Work out the finished part from the listing and answer in its coordinate system (mm). A direction names the side the tool comes from. Round coordinates to 2 decimals unless told otherwise and drop trailing zeros. Write each loop counter-clockwise with the first axis right and the second up, starting at its lowest first coordinate (ties: lowest second). Pieces come first, ordered by that corner, then holes.
1. Find section B-B (y = 3.75). Write down the section's boundary in (x, z).
2. Flat-ended cylindrical pins translate along their axes: pin 1 Ø0.6 at (x, z) = (-7.5, 0) entering from -Y; pin 2 Ø0.6 at (x, z) = (-6, -0.5) entering from +Y. Find the tip coordinate at first contact, or state that the pin passes through.
3. Find section D-D (y = 0). Write down the section's boundary in (x, z), and give its area (3 significant figures).
4. Find section C-C (z = 0.2). Write down the section's boundary in (x, y), and give its area (3 significant figures).
5. Find section A-A (x = 0). Write down the section's boundary in (y, z).
6. Determine the mould class of faces 1 (the face through (4, 0, 1)), 2 (the face through (0, 6, 0)), 3 (the face through (10, 0, 0)) for opening direction Y: pulls with the +Y half, pulls with the -Y half, needs draft (parallel to the pull), parting line crosses it, or undercut.
7. A tool of negligible diameter and unlimited length cuts with its end or side. For faces 4 (the face through (4, 0, -1)), 5 (the face through (3.37, 0, 0)), 6 (the face through (-6, 3.37, 0)), from which of +Z, -Z, +X, -X, +Y, -Y can it reach the whole face along a straight path? Write none if from no direction.
8. Straight lines are drawn through the part: probe 1 along Y at (x, z) = (-3, -0.55); probe 2 along Y at (x, z) = (-6, 0); probe 3 along X at (y, z) = (4, -0.2). For each, find the intervals that lie inside material, in ascending order.
```python
from build123d import *

# Parameters (mm, degrees)
SCHIZZO1_R                   = 10
ESTRUSIONE_ESTRUSIONE1_DEPTH = 1
TAGLIO_ESTRUSIONE1_DEPTH     = 15.282856857


with BuildPart() as part:
    # Schizzo1 → Estrusione-Estrusione1 (new, symmetric)
    with BuildSketch(Plane.XY):
        Circle(SCHIZZO1_R)
    extrude(amount=ESTRUSIONE_ESTRUSIONE1_DEPTH, both=True)

    # Schizzo2 → Taglio-Estrusione1 (cut, through all)
    with BuildSketch(Plane.XY.offset(1)):
        with BuildLine():
            Line((-3.37, -3.37), (-3.37, 3.37))
            Line((-3.37, 3.37), (-9.415046468, 3.37))
            ThreePointArc((-9.415046468, 3.37), (-10, 0), (-9.415046468, -3.37))
            Line((-9.415046468, -3.37), (-3.37, -3.37))
        make_face()
        with BuildLine():
            Line((-3.37, 4.964181705), (-3.37, -4.964181705))
            ThreePointArc((-3.37, -4.964181705), (0, -6), (3.37, -4.964181705))
            Line((3.37, -4.964181705), (3.37, 4.964181705))
            ThreePointArc((3.37, 4.964181705), (0, 6), (-3.37, 4.964181705))
        make_face()
    extrude(amount=-TAGLIO_ESTRUSIONE1_DEPTH, mode=Mode.SUBTRACT)


solid = part.part
```
Worked answers:
1. outline: (-9.27, -1) - (-3.37, -1) - (-3.37, 1) - (-9.27, 1) - close; (3.37, -1) - (9.27, -1) - (9.27, 1) - (3.37, 1) - close
2. pin 1: stops at y = -6.94
2. pin 2: stops at y = 8.22
3. outline: (3.37, -1) - (10, -1) - (10, 1) - (3.37, 1) - close
3. area: 13.3 mm2
4. outline: (-9.42, -3.37) arc R10 ccw (long way) to (-9.42, 3.37) - (-3.37, 3.37) - (-3.37, 4.96) arc R6 cw to (3.37, 4.96) - (3.37, -4.96) arc R6 cw to (-3.37, -4.96) - (-3.37, -3.37) - close
4. area: 194 mm2
5. outline: (-10, -1) - (-6, -1) - (-6, 1) - (-10, 1) - close; (6, -1) - (10, -1) - (10, 1) - (6, 1) - close
6. face 1: needs draft
6. face 2: undercut
6. face 3: parting line crosses it
7. face 4: -Z, +X, -X, +Y, -Y
7. face 5: +Z, -Z
7. face 6: +Z, -Z, -X
8. probe 1: y = -9.54 to -5.2, 5.2 to 9.54
8. probe 2: y = -8 to -3.37, 3.37 to 8
8. probe 3: x = -9.17 to -3.37, 3.37 to 9.17
